Can you work these out from the drawing? Everything is in mm from the part's minimum corner. A direction names the side the tool comes from. Give positions to 0.01 mm unless a question says otherwise; leave off trailing zeros. Loops run counter-clockwise (first coordinate to the right, second up) from the corner with the lowest first, then second, coordinate; pieces in that order, holes last. Notation, with made-up numbers: (-36.75, 59.5) -> (3.25, 59.5) arc R10 cw to (3.25, 76.5) -> close; hole circle Ø11 at (22.5, -5). An arc over 180 degrees is marked (long way). Return JSON: item names as keys, results as strings. Group by question number.
Q1. Suppose I cut it at B-B, the plane z = 27. Please give me the cut outline in (x, y).
Q2. Suppose I cut it at C-C, the plane z = 10.49. Please give me the cut outline in (x, y).
Q3. Thinking about a two-plate mould opening in Z: for the marked faces 1, 2 and 3, which applies, pulls with the +Z half, pulls with the -Z half, needs draft (parallel to the pull), parting line crosses it, or undercut?
Q4. Suppose I cut it at A-A, the plane x = 27. Please give me the cut outline in (y, z).
Q5. Will these pins go through, and if not, where does the flat tip stop? pin 1 (10 mm diameter, centred on x = 9.5, y = 15.5, fed in from -Z); pin 2 (1 mm diameter, centred on y = 23.5, z = 28.5, fed in from -X); pin 3 (6 mm diameter, centred on y = 11.5, z = 40, fed in from +X).
Q6. I need wall thicknesses on line 1 along Y through (x, z) = (10.5, 7.5); line 2 along Z through (x, y) = (27.5, 12); line 3 along X through (y, z) = (16.5, 10.49). Which ranges of each line are inside material? Lowest first, please. Write a range as [from, to].
Q7. Suppose I cut it at D-D, the plane y = 16.5. Please give me the cut outline in (x, z) (3 decimals).
Q8. Which directions (+Z, -Z, +X, -X, +Y, -Y) give clear straight access to the entire face, cutting with the end or side of a thin tool? Please do the marked faces 4 and 5.
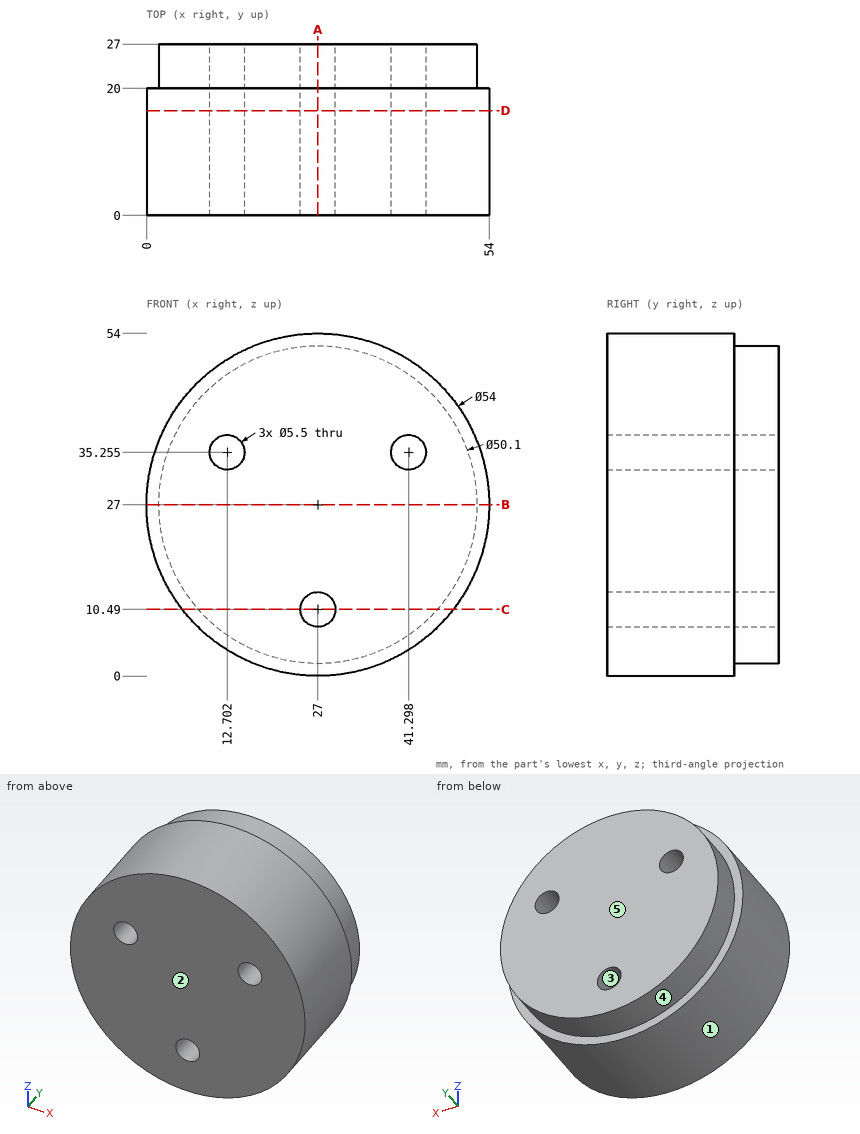
Ans:
{
 "1": {"outline": "(0, 0) -> (54, 0) -> (54, 20) -> (52.05, 20) -> (52.05, 27) -> (1.95, 27) -> (1.95, 20) -> (0, 20) -> close"},
 "2": {"outline": "(5.64, 0) -> (24.25, 0) -> (24.25, 27) -> (8.16, 27) -> (8.16, 20) -> (5.64, 20) -> close; (29.75, 0) -> (48.36, 0) -> (48.36, 20) -> (45.84, 20) -> (45.84, 27) -> (29.75, 27) -> close"},
 "3": {"face 1": "parting line crosses it", "face 2": "needs draft", "face 3": "undercut"},
 "4": {"outline": "(0, 0) -> (20, 0) -> (20, 1.95) -> (27, 1.95) -> (27, 7.74) -> (0, 7.74) -> close; (0, 13.24) -> (27, 13.24) -> (27, 52.05) -> (20, 52.05) -> (20, 54) -> (0, 54) -> close"},
 "5": {"pin 1": "stops at z = 3.07", "pin 2": "stops at x = 1.97", "pin 3": "stops at x = 52.08"},
 "6": {"line 1": "y = [0, 20]", "line 2": "z = [0, 7.79], [13.19, 54]", "line 3": "x = [5.64, 24.25], [29.75, 48.36]"},
 "7": {"outline": "circle Ø54 at (27, 27); hole circle Ø5.5 at (12.702, 35.255); hole circle Ø5.5 at (27, 10.49); hole circle Ø5.5 at (41.298, 35.255)"},
 "8": {"face 4": "+Y", "face 5": "+Z, -Z, +X, -X, +Y"}
}
